Can you work these out from the model? Positions are in its coordinate system, mm. Face numbers are marked on the shaded views. Round coordinates to 2 decimals unless told otherwise and drop trailing zeros. Write each loop counter-clockwise with the first axis right and the second up, starting at its lowest first coordinate (ties: lowest second). Pieces come first, ordered by that corner, then holes. Notation, with made-up numbers: M 18,27.25 L 36,27.25 A14 ccw 36,33.25 Z; hole C -11,61 d10. An arc over 180 degrees is marked long. Answer as a JSON object with one key per item and string values. Group by question number.
1) Please list where these lines run through material, in increasing order: L1, parallel to Z at x = 8.5, y = 0; L2, parallel to X at y = 27, z = 481.5; L3, parallel to Z at x = -153, y = 153. Write a range as [from, to].
2) I'm going to push flat-ended pins straight in: pin 1 Ø1 at (x, z) = (317, -18) entering from +Y; pin 2 Ø1 at (x, y) = (226.5, 288) entering from +Z; pin 3 Ø5 at (y, z) = (75.5, 684.5) entering from -X. Where does each tip first touch, or does it pass through?
3) Suppose I cut it at A-A, the plane y = 0. Write out the boundary of the cut face in (x, z), and give its area (3 significant figures).
4) Suppose I cut it at B-B, the plane x = 26. Write out the boundary of the cut face in (y, z).
5) If we mould it in two halves opening along Y, with no side actions, what happens to the marked faces 1, 2 and 3? For each: +Y half, -Y half, draft (parallel to the pull), parting line (faces both ways), or undercut.
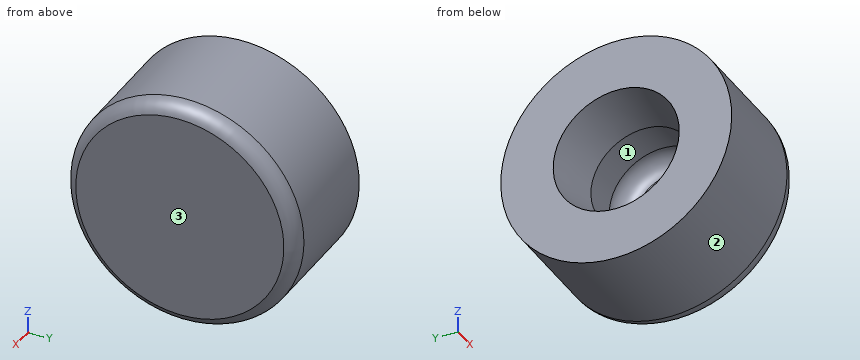
from build123d import *


with BuildPart() as f1:
    # F0 (on Front) → F1 (revolve)
    with BuildSketch(Plane.XZ):
        with BuildLine():
            Line((-51.01523, 28.884935), (-424.153769, -48.112668))
            Line((-424.153769, -48.112668), (-424.153769, -429.112668))
            Line((-424.153769, -429.112668), (337.846231, -429.112668))
            ThreePointArc((337.846231, -429.112668), (410.449368, -406.313361), (456.98477, -346.1014))
            Line((456.98477, -346.1014), (456.98477, 409.884935))
            Line((456.98477, 409.884935), (329.98477, 409.884935))
            Line((329.98477, 409.884935), (329.98477, 155.884935))
            ThreePointArc((329.98477, 155.884935), (292.787331, 66.082374), (202.98477, 28.884935))
            Line((202.98477, 28.884935), (-51.01523, 28.884935))
        make_face()
    revolve(axis=Axis((393.48477, 0, 409.884935), (-1, 0, 0)))


solid = f1.part
Results:
{
 "1": {"L1": "[-429.11, 28.88], [790.88, 1248.88]", "L2": "[329.98, 456.98]", "L3": "[-415.04, 38.09], [781.68, 1234.81]"},
 "2": {"pin 1": "y = 721.98", "pin 2": "z = 1198.09", "pin 3": "x = 325.54"},
 "3": {"outline": "M -424.15,-429.11 L 337.85,-429.11 A127 ccw 456.98,-346.1 L 456.98,1165.87 A127 ccw 337.85,1248.88 L -424.15,1248.88 L -424.15,867.88 L -51.02,790.88 L 202.98,790.88 A127 cw 329.98,663.88 L 329.98,155.88 A127 cw 202.98,28.88 L -51.02,28.88 L -424.15,-48.11 Z", "area": "877,000 mm^2"},
 "4": {"outline": "C 0,409.88 d1678; hole C 0,409.88 d762"},
 "5": {"face 1": "undercut", "face 2": "parting line", "face 3": "draft"}
}
